Input: part model. Units: mm. Frame: model coordinates. A direction names the side the tool comes from. Give positions to 0.01 mm unless a question says otherwise; leave off trailing zeros. Loops run counter-clockwise (first coordinate to the right, second up) from the corner with the lowest first, then second, coordinate; pieces in that order, holes last. Notation, with made-up numbers: (-29, 8) -> (22, 8) arc R26 ccw to (22, 25) -> close; hole circle Ø1 at (-14.75, 42). An arc over 180 degrees is marked (long way). Answer as a JSON object with one key per item and string values. Group by question number.
```python
from build123d import *
from OCP.BRepFilletAPI import BRepFilletAPI_MakeChamfer

# Parameters (mm, degrees)
ESQUISSE1_W             = 192.96
ESQUISSE1_H             = 110.76
C_VITRE_DEPTH           = 0.82
CONG_1_R                = 7.88
ESQUISSE2_W             = 171.38
ESQUISSE2_H             = 96.96
C_TOUCH_DEPTH           = 0.8
ESQUISSE3_W             = 166.2
ESQUISSE3_H             = 100.6
BOSS_EXTRU_3_DEPTH      = 4.58
ESQUISSE4_W             = 15
ESQUISSE4_H             = 8
ESQUISSE4_R             = 1.5
ESQUISSE4_W_2           = 8
ESQUISSE4_H_2           = 15
ESQUISSE4_R_2           = 1.25
BOSS_EXTRU_4_DEPTH      = 2.5
CHANFREIN1_SIZE         = 2.5
CHANFREIN1_SIZE_2       = 4.5
BOSS_EXTRU_5_DEPTH      = 0.5
CONG_2_R                = 0.5
ENL_V_MAT_EXTRU_1_DEPTH = 133.991041409
ENL_V_MAT_EXTRU_2_REACH = 149.027
ENL_V_MAT_EXTRU_3_REACH = 149.027


with BuildPart() as part:
    # Esquisse1 → c_vitre (new body)
    with BuildSketch(Plane.XY):
        Rectangle(ESQUISSE1_W, ESQUISSE1_H)
    extrude(amount=C_VITRE_DEPTH)

    # Congé1
    cong_1_edges = [part.edges().sort_by_distance(p)[0] for p in [
        (-96.48, 55.38, 0.41),
        (96.48, 55.38, 0.41),
        (96.48, -55.38, 0.41),
        (-96.48, -55.38, 0.41),
    ]]
    fillet(cong_1_edges, radius=CONG_1_R)

    # Esquisse2 → c_touch (add)
    with BuildSketch(Plane(origin=(0, 0, 0), x_dir=(-1, 0, 0), z_dir=(0, 0, -1))):
        with Locations((5.81, -0.58)):
            Rectangle(ESQUISSE2_W, ESQUISSE2_H)
    extrude(amount=C_TOUCH_DEPTH)

    # Esquisse3 → Boss.-Extru.3 (add)
    with BuildSketch(Plane(origin=(0, 0, -0.8), x_dir=(-1, 0, 0), z_dir=(0, 0, -1))):
        with Locations((-1.49, -1.55)):
            Rectangle(ESQUISSE3_W, ESQUISSE3_H)
    extrude(amount=BOSS_EXTRU_3_DEPTH)

    # Esquisse4 → Boss.-Extru.4 (add)
    # profile 1 of 8: a face of its own
    with BuildSketch(Plane(origin=(0, 0, -5.38), x_dir=(-1, 0, 0), z_dir=(0, 0, -1))):
        with Locations((-64.59, 33.8)):
            Rectangle(ESQUISSE4_W, ESQUISSE4_H)
        with Locations((-64.59, 33.8)):
            Circle(ESQUISSE4_R, mode=Mode.SUBTRACT)
    # profile 2 of 8: a face of its own
    with BuildSketch(Plane(origin=(0, 0, -5.38), x_dir=(-1, 0, 0), z_dir=(0, 0, -1))):
        with Locations((-64.59, -31.812830284)):
            Rectangle(ESQUISSE4_W, ESQUISSE4_H)
        with Locations((-64.59, -31.812830284)):
            Circle(ESQUISSE4_R, mode=Mode.SUBTRACT)
    # profile 3 of 8: a face of its own
    with BuildSketch(Plane(origin=(0, 0, -5.38), x_dir=(-1, 0, 0), z_dir=(0, 0, -1))):
        with Locations((61.61, -31.812830284)):
            Rectangle(ESQUISSE4_W, ESQUISSE4_H)
        with Locations((61.61, -31.812830284)):
            Circle(ESQUISSE4_R, mode=Mode.SUBTRACT)
    # profile 4 of 8: a face of its own
    with BuildSketch(Plane(origin=(0, 0, -5.38), x_dir=(-1, 0, 0), z_dir=(0, 0, -1))):
        with Locations((61.61, 33.837169716)):
            Rectangle(ESQUISSE4_W, ESQUISSE4_H)
        with Locations((61.61, 33.837169716)):
            Circle(ESQUISSE4_R, mode=Mode.SUBTRACT)
    # profile 5 of 8: a face of its own
    with BuildSketch(Plane(origin=(0, 0, -5.38), x_dir=(-1, 0, 0), z_dir=(0, 0, -1))):
        with Locations((-35.49, 27.95)):
            Rectangle(ESQUISSE4_W_2, ESQUISSE4_H_2)
        with Locations((-35.49, 27.95)):
            Circle(ESQUISSE4_R_2, mode=Mode.SUBTRACT)
    # profile 6 of 8: a face of its own
    with BuildSketch(Plane(origin=(0, 0, -5.38), x_dir=(-1, 0, 0), z_dir=(0, 0, -1))):
        with Locations((-35.49, -21.05)):
            Rectangle(ESQUISSE4_W_2, ESQUISSE4_H_2)
        with Locations((-35.49, -21.05)):
            Circle(ESQUISSE4_R_2, mode=Mode.SUBTRACT)
    # profile 7 of 8: a face of its own
    with BuildSketch(Plane(origin=(0, 0, -5.38), x_dir=(-1, 0, 0), z_dir=(0, 0, -1))):
        with Locations((22.51, -21.05)):
            Rectangle(ESQUISSE4_W_2, ESQUISSE4_H_2)
        with Locations((22.51, -21.05)):
            Circle(ESQUISSE4_R_2, mode=Mode.SUBTRACT)
    # profile 8 of 8: a face of its own
    with BuildSketch(Plane(origin=(0, 0, -5.38), x_dir=(-1, 0, 0), z_dir=(0, 0, -1))):
        with Locations((22.51, 27.95)):
            Rectangle(ESQUISSE4_W_2, ESQUISSE4_H_2)
        with Locations((22.51, 27.95)):
            Circle(ESQUISSE4_R_2, mode=Mode.SUBTRACT)
    extrude(amount=BOSS_EXTRU_4_DEPTH)

    # Chanfrein1
    chanfrein1_edges_1 = [part.edges().sort_by_distance(p)[0] for p in [
        (-69.11, -31.812830284, -7.88),
    ]]
    chanfrein1_side_1 = [part.faces().sort_by_distance(p)[0] for p in [
        (-69.11, -31.812830284, -7.83),
    ]]
    chanfrein1_edges_2 = [part.edges().sort_by_distance(p)[0] for p in [
        (-54.11, -31.812830284, -7.88),
    ]]
    chanfrein1_side_2 = [part.faces().sort_by_distance(p)[0] for p in [
        (-54.11, -31.812830284, -7.83),
    ]]
    chanfrein1_edges_3 = [part.edges().sort_by_distance(p)[0] for p in [
        (-22.51, -28.55, -7.88),
    ]]
    chanfrein1_side_3 = [part.faces().sort_by_distance(p)[0] for p in [
        (-22.51, -28.55, -7.83),
    ]]
    chanfrein1_edges_4 = [part.edges().sort_by_distance(p)[0] for p in [
        (-22.51, -13.55, -7.88),
    ]]
    chanfrein1_side_4 = [part.faces().sort_by_distance(p)[0] for p in [
        (-22.51, -13.55, -7.83),
    ]]
    chanfrein1_edges_5 = [part.edges().sort_by_distance(p)[0] for p in [
        (-69.11, 33.837169716, -7.88),
    ]]
    chanfrein1_side_5 = [part.faces().sort_by_distance(p)[0] for p in [
        (-69.11, 33.837169716, -7.83),
    ]]
    chanfrein1_edges_6 = [part.edges().sort_by_distance(p)[0] for p in [
        (-54.11, 33.837169716, -7.88),
    ]]
    chanfrein1_side_6 = [part.faces().sort_by_distance(p)[0] for p in [
        (-54.11, 33.837169716, -7.83),
    ]]
    chanfrein1_edges_7 = [part.edges().sort_by_distance(p)[0] for p in [
        (-22.51, 20.45, -7.88),
    ]]
    chanfrein1_side_7 = [part.faces().sort_by_distance(p)[0] for p in [
        (-22.51, 20.45, -7.83),
    ]]
    chanfrein1_edges_8 = [part.edges().sort_by_distance(p)[0] for p in [
        (-22.51, 35.45, -7.88),
    ]]
    chanfrein1_side_8 = [part.faces().sort_by_distance(p)[0] for p in [
        (-22.51, 35.45, -7.83),
    ]]
    chanfrein1_edges_9 = [part.edges().sort_by_distance(p)[0] for p in [
        (35.49, 35.45, -7.88),
    ]]
    chanfrein1_side_9 = [part.faces().sort_by_distance(p)[0] for p in [
        (35.49, 35.45, -7.83),
    ]]
    chanfrein1_edges_10 = [part.edges().sort_by_distance(p)[0] for p in [
        (57.09, 33.8, -7.88),
    ]]
    chanfrein1_side_10 = [part.faces().sort_by_distance(p)[0] for p in [
        (57.09, 33.8, -7.83),
    ]]
    chanfrein1_edges_11 = [part.edges().sort_by_distance(p)[0] for p in [
        (72.09, 33.8, -7.88),
    ]]
    chanfrein1_side_11 = [part.faces().sort_by_distance(p)[0] for p in [
        (72.09, 33.8, -7.83),
    ]]
    chanfrein1_edges_12 = [part.edges().sort_by_distance(p)[0] for p in [
        (35.49, 20.45, -7.88),
    ]]
    chanfrein1_side_12 = [part.faces().sort_by_distance(p)[0] for p in [
        (35.49, 20.45, -7.83),
    ]]
    chanfrein1_edges_13 = [part.edges().sort_by_distance(p)[0] for p in [
        (35.49, -13.55, -7.88),
    ]]
    chanfrein1_side_13 = [part.faces().sort_by_distance(p)[0] for p in [
        (35.49, -13.55, -7.83),
    ]]
    chanfrein1_edges_14 = [part.edges().sort_by_distance(p)[0] for p in [
        (35.49, -28.55, -7.88),
    ]]
    chanfrein1_side_14 = [part.faces().sort_by_distance(p)[0] for p in [
        (35.49, -28.55, -7.83),
    ]]
    chanfrein1_edges_15 = [part.edges().sort_by_distance(p)[0] for p in [
        (57.09, -31.812830284, -7.88),
    ]]
    chanfrein1_side_15 = [part.faces().sort_by_distance(p)[0] for p in [
        (57.09, -31.812830284, -7.83),
    ]]
    chanfrein1_edges_16 = [part.edges().sort_by_distance(p)[0] for p in [
        (72.09, -31.812830284, -7.88),
    ]]
    chanfrein1_side_16 = [part.faces().sort_by_distance(p)[0] for p in [
        (72.09, -31.812830284, -7.83),
    ]]
    chanfrein1 = BRepFilletAPI_MakeChamfer(part.part.solid().wrapped)
    for e in chanfrein1_edges_1:
        chanfrein1.Add(CHANFREIN1_SIZE - 0.0001, CHANFREIN1_SIZE_2 - 0.0001, e.wrapped, chanfrein1_side_1[0].wrapped)
    for e in chanfrein1_edges_2:
        chanfrein1.Add(CHANFREIN1_SIZE - 0.0001, CHANFREIN1_SIZE_2 - 0.0001, e.wrapped, chanfrein1_side_2[0].wrapped)
    for e in chanfrein1_edges_3:
        chanfrein1.Add(CHANFREIN1_SIZE - 0.0001, CHANFREIN1_SIZE_2 - 0.0001, e.wrapped, chanfrein1_side_3[0].wrapped)
    for e in chanfrein1_edges_4:
        chanfrein1.Add(CHANFREIN1_SIZE - 0.0001, CHANFREIN1_SIZE_2 - 0.0001, e.wrapped, chanfrein1_side_4[0].wrapped)
    for e in chanfrein1_edges_5:
        chanfrein1.Add(CHANFREIN1_SIZE - 0.0001, CHANFREIN1_SIZE_2 - 0.0001, e.wrapped, chanfrein1_side_5[0].wrapped)
    for e in chanfrein1_edges_6:
        chanfrein1.Add(CHANFREIN1_SIZE - 0.0001, CHANFREIN1_SIZE_2 - 0.0001, e.wrapped, chanfrein1_side_6[0].wrapped)
    for e in chanfrein1_edges_7:
        chanfrein1.Add(CHANFREIN1_SIZE - 0.0001, CHANFREIN1_SIZE_2 - 0.0001, e.wrapped, chanfrein1_side_7[0].wrapped)
    for e in chanfrein1_edges_8:
        chanfrein1.Add(CHANFREIN1_SIZE - 0.0001, CHANFREIN1_SIZE_2 - 0.0001, e.wrapped, chanfrein1_side_8[0].wrapped)
    for e in chanfrein1_edges_9:
        chanfrein1.Add(CHANFREIN1_SIZE - 0.0001, CHANFREIN1_SIZE_2 - 0.0001, e.wrapped, chanfrein1_side_9[0].wrapped)
    for e in chanfrein1_edges_10:
        chanfrein1.Add(CHANFREIN1_SIZE - 0.0001, CHANFREIN1_SIZE_2 - 0.0001, e.wrapped, chanfrein1_side_10[0].wrapped)
    for e in chanfrein1_edges_11:
        chanfrein1.Add(CHANFREIN1_SIZE - 0.0001, CHANFREIN1_SIZE_2 - 0.0001, e.wrapped, chanfrein1_side_11[0].wrapped)
    for e in chanfrein1_edges_12:
        chanfrein1.Add(CHANFREIN1_SIZE - 0.0001, CHANFREIN1_SIZE_2 - 0.0001, e.wrapped, chanfrein1_side_12[0].wrapped)
    for e in chanfrein1_edges_13:
        chanfrein1.Add(CHANFREIN1_SIZE - 0.0001, CHANFREIN1_SIZE_2 - 0.0001, e.wrapped, chanfrein1_side_13[0].wrapped)
    for e in chanfrein1_edges_14:
        chanfrein1.Add(CHANFREIN1_SIZE - 0.0001, CHANFREIN1_SIZE_2 - 0.0001, e.wrapped, chanfrein1_side_14[0].wrapped)
    for e in chanfrein1_edges_15:
        chanfrein1.Add(CHANFREIN1_SIZE - 0.0001, CHANFREIN1_SIZE_2 - 0.0001, e.wrapped, chanfrein1_side_15[0].wrapped)
    for e in chanfrein1_edges_16:
        chanfrein1.Add(CHANFREIN1_SIZE - 0.0001, CHANFREIN1_SIZE_2 - 0.0001, e.wrapped, chanfrein1_side_16[0].wrapped)
    add(Compound.cast(chanfrein1.Shape()), mode=Mode.REPLACE)  # a hair under: the kernel refuses the full size

    # Esquisse5 → Boss.-Extru.5 (add)
    with BuildSketch(Plane(origin=(0, 0, -5.38), x_dir=(-1, 0, 0), z_dir=(0, 0, -1))):
        with BuildLine():
            Line((47.51, 45.85), (-50.49, 45.85))
            ThreePointArc((-50.49, 45.85), (-51.99, 44.35), (-50.49, 42.85))
            Line((-50.49, 42.85), (47.51, 42.85))
            ThreePointArc((47.51, 42.85), (49.01, 44.35), (47.51, 45.85))
        make_face()
        with BuildLine():
            Line((27.51, -43.85), (-30.49, -43.85))
            ThreePointArc((-30.49, -43.85), (-31.99, -45.35), (-30.49, -46.85))
            Line((-30.49, -46.85), (27.51, -46.85))
            ThreePointArc((27.51, -46.85), (29.01, -45.35), (27.51, -43.85))
        make_face()
    extrude(amount=BOSS_EXTRU_5_DEPTH)

    # Congé2
    cong_2_edges = [part.edges().sort_by_distance(p)[0] for p in [
        (1.49, 42.85, -5.88),
        (51.99, 44.35, -5.88),
        (1.49, 45.85, -5.88),
        (1.49, -46.85, -5.88),
        (31.99, -45.35, -5.88),
        (1.49, -43.85, -5.88),
        (-49.01, 44.35, -5.88),
        (-29.01, -45.35, -5.88),
    ]]
    fillet(cong_2_edges, radius=CONG_2_R - 0.0001)  # a hair under: the kernel refuses the full size

    # Esquisse7 → Enlèv. mat.-Extru.1 (cut, through all)
    with BuildSketch(Plane.XZ.offset(35.812830284)):
        Polygon((58.737300823, -5.38), (70.442699177, -5.38), (67.382699177, -7.08), (61.797300823, -7.08), align=None)
        Polygon((-67.462699177, -5.38), (-64.402699177, -7.08), (-58.817300823, -7.08), (-55.757300823, -5.38), align=None)
    extrude(amount=-ENL_V_MAT_EXTRU_1_DEPTH, mode=Mode.SUBTRACT)

    # Enlèv. mat.-Extru.2: up to this face of the body (flat: up to its plane)
    enl_v_mat_extru_2_end = Plane(part.part.faces().sort_by_distance((-26.51, -21.05, -6.451430159))[0])
    # Esquisse8 → Enlèv. mat.-Extru.2 (cut, up to the picked face)
    with BuildSketch(Plane(origin=(39.49, 0, 0), x_dir=(0, 0, -1), z_dir=(1, 0, 0)), mode=Mode.PRIVATE) as enl_v_mat_extru_2_sk1:
        Polygon((5.38, -15.197300823), (5.38, -26.902699177), (7.08, -23.842699177), (7.08, -18.257300823), align=None)
    enl_v_mat_extru_2_tool1 = split(extrude(enl_v_mat_extru_2_sk1.sketch, amount=-ENL_V_MAT_EXTRU_2_REACH, mode=Mode.PRIVATE), bisect_by=enl_v_mat_extru_2_end, keep=Keep.BOTH, mode=Mode.PRIVATE)
    add(enl_v_mat_extru_2_tool1.solids().sort_by(Axis((39.49, -21.05, -6.129715), (-1, 0, 0)))[0], mode=Mode.SUBTRACT)

    # Enlèv. mat.-Extru.3: up to this face of the body (flat: up to its plane)
    enl_v_mat_extru_3_end = Plane(part.part.faces().sort_by_distance((-26.51, 27.95, -6.451430159))[0])
    # Esquisse9 → Enlèv. mat.-Extru.3 (cut, up to the picked face)
    with BuildSketch(Plane(origin=(39.49, 0, 0), x_dir=(0, 0, -1), z_dir=(1, 0, 0)), mode=Mode.PRIVATE) as enl_v_mat_extru_3_sk1:
        Polygon((5.38, 22.097300823), (5.38, 33.802699177), (7.08, 30.742699177), (7.08, 25.157300823), align=None)
    enl_v_mat_extru_3_tool1 = split(extrude(enl_v_mat_extru_3_sk1.sketch, amount=-ENL_V_MAT_EXTRU_3_REACH, mode=Mode.PRIVATE), bisect_by=enl_v_mat_extru_3_end, keep=Keep.BOTH, mode=Mode.PRIVATE)
    add(enl_v_mat_extru_3_tool1.solids().sort_by(Axis((39.49, 27.95, -6.129715), (-1, 0, 0)))[0], mode=Mode.SUBTRACT)


solid = part.part
```
Q1. Ray query, probe 1 along X at (y, z) = (27.95, -7.25); probe 2 along Y at (x, z) = (64.59, -7.35); probe 3 along Z at (x, y) = (80.5, -39.5). Return the intervals inside material, ascending.
Q2. Section B-B on y = 10. Return the cut outline in (x, z), then the cut area to 3 significant figures.
Q3. Pull-direction query (X, two-part tool) for faces 5 (the face through (94.11, -53.133, 0.416)), 6 (the face through (34.7, -22.3, -7.08)), 7 (the face through (-66.829, -31.869, -6.648)), 8 (the face through (34.7, 29.2, -7.08)); classes: +X half, -X half, draft (parallel to the pull), parting line (faces both ways), or undercut.
Q4. Section C-C on z = -3. Return the cut outline in (x, y).
Q5. Set-up query: faces 1 (the face through (-22.454, 22.731, -6.648)), 2 (the face through (-56.391, 33.781, -6.648)), 3 (the face through (-63, 35, -7.08)), 4 (the face through (3, -51.85, -3)). Return all of +Z, -Z, +X, -X, +Y, -Y with unobstructed straight access to the full face (end or side cutting, diameter ignored); none if empty.
Q6. Section D-D on x = -78. Return the cut outline in (y, z), then the cut area to 3 significant figures.
Q7. Pin query (flat end, axial travel): pin 1 Ø5 at (x, z) = (30.5, -3.5) entering from -Y; pin 2 Ø1.4 at (x, z) = (-8.5, -3.5) entering from +Y; pin 3 Ø2 at (x, y) = (3.5, 44) entering from -Z. Return the tip coordinate at first contact, or that it passes through.
Numbers:
{
 "1": {"probe 1": "x = -26.51 to -23.76, -21.26 to -18.51, 31.49 to 34.24, 36.74 to 39.49", "probe 2": "y = -35.81 to -33.31, -30.31 to -27.81, 29.8 to 32.3, 35.3 to 37.8", "probe 3": "z = -5.38 to -0.8, 0 to 0.82"},
 "2": {"outline": "(-96.48, 0) -> (-91.5, 0) -> (-91.5, -0.8) -> (-81.61, -0.8) -> (-81.61, -5.38) -> (84.59, -5.38) -> (84.59, -0.8) -> (79.88, -0.8) -> (79.88, 0) -> (96.48, 0) -> (96.48, 0.82) -> (-96.48, 0.82) -> close", "area": "1,060 mm²"},
 "3": {"face 5": "+X half", "face 6": "draft", "face 7": "-X half", "face 8": "undercut"},
 "4": {"outline": "(-81.61, -51.85) -> (84.59, -51.85) -> (84.59, 48.75) -> (-81.61, 48.75) -> close"},
 "5": {"face 1": "-Z, +X, -X", "face 2": "-Z, +Y, -Y", "face 3": "+Y, -Y", "face 4": "-Z, +X, -X, -Y"},
 "6": {"outline": "(-55.38, 0) -> (-49.06, 0) -> (-49.06, -0.8) -> (-51.85, -0.8) -> (-51.85, -5.38) -> (48.75, -5.38) -> (48.75, -0.8) -> (47.9, -0.8) -> (47.9, 0) -> (55.38, 0) -> (55.38, 0.82) -> (-55.38, 0.82) -> close", "area": "629 mm²"},
 "7": {"pin 1": "stops at y = -51.85", "pin 2": "stops at y = 48.75", "pin 3": "stops at z = -5.88"}
}
